Design review of the part shown in the three views and the two pictorial views. Dimensions are in mm from the part's minimum x, y and z. A direction names the side the tool comes from. Give positions to 0.01 mm unless a question says otherwise; leave off trailing zeros. Loops run counter-clockwise (first coordinate to the right, second up) from the corner with the lowest first, then second, coordinate; pieces in that order, holes last. Notation, with made-up numbers: (-2.5, 55.25) - (22.5, 55.25) arc R26 cw to (22.5, 87.25) - close; hole circle Ø1 at (-15, -5.5). An arc over 180 degrees is marked (long way). Return JSON: item names as keys, results as strings. Group by question number.
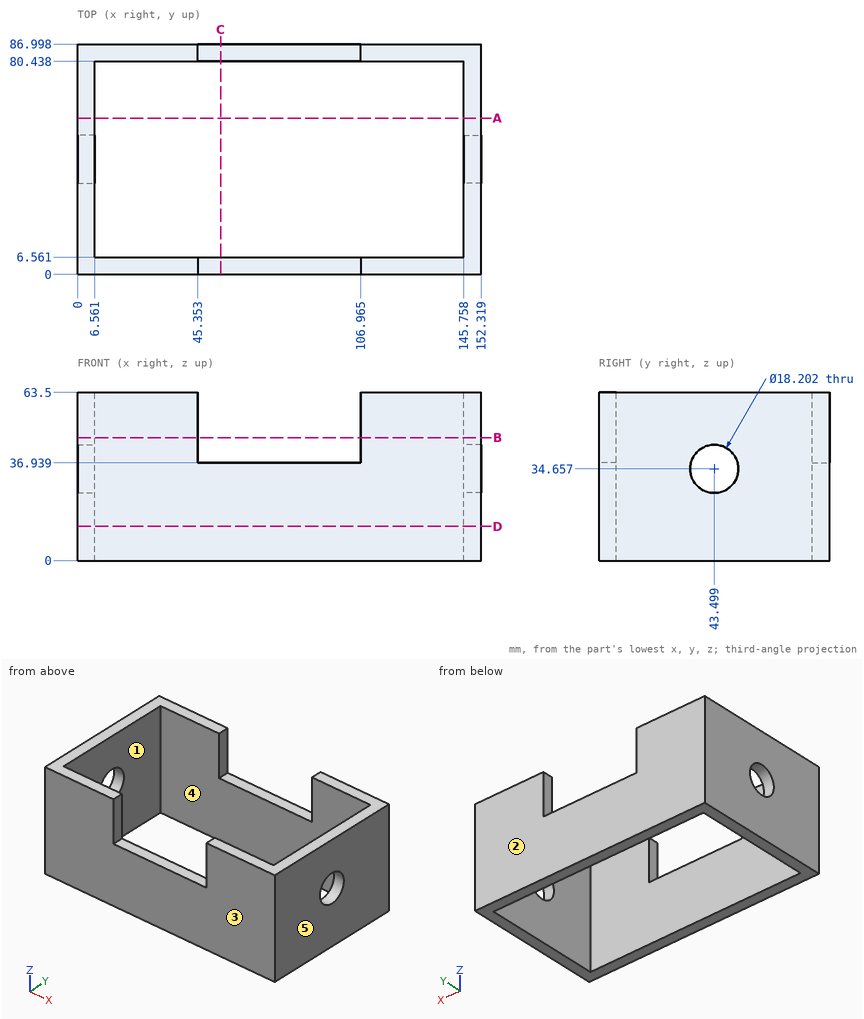
Item 1: Take a section at C-C (x = 54). State the section outline as (y, z) points.
Item 2: Mouldability with a two-part tool opening along Y and no side actions: class the marked faces 1, 2 and 3 as +Y half, -Y half, draft (parallel to the pull), parting line (faces both ways), or undercut.
Item 3: Tool access review of the marked faces 4 and 5: name each direction out of +Z, -Z, +X, -X, +Y, -Y from which nothing blocks a thin tool from reaching the whole face with its end or side.
Item 4: Take a section at B-B (z = 46.5). State the section outline as (x, y) points (1 decimal), then the cut area to 3 significant figures.
Item 5: Take a section at D-D (z = 13). State the section outline as (x, y) points, then the cut area to 3 significant figures.
Item 6: Take a section at A-A (y = 59). State the section outline as (x, z) points, then the cut area to 3 significant figures.
Item 7: For L1, parallel to Y at x = 61, z = 21.5; L2, parallel to X at y = 63, z = 34.5; L3, parallel to Z at x = 60, y = 83, list the stretches that pass through material, from the lowest coordinate up. Write a range as from..to.
Item 8: For P1, Ø10, axis at x = 75, y = 73, coming from the -Z side; P2, Ø5, axis at x = 71.5, y = 2.5, coming from the +Z side, all flat-tipped, find the tip position at first contact; note any pin that passes through.
Check sheet entries:
{
 "1": {"outline": "(0, 0) - (6.56, 0) - (6.56, 36.94) - (0, 36.94) - close; (80.44, 0) - (87, 0) - (87, 36.94) - (80.44, 36.94) - close"},
 "2": {"face 1": "undercut", "face 2": "+Y half", "face 3": "-Y half"},
 "3": {"face 4": "+Z, -Z", "face 5": "+Z, -Z, +X, +Y, -Y"},
 "4": {"outline": "(0, 0) - (45.4, 0) - (45.4, 6.6) - (6.6, 6.6) - (6.6, 80.4) - (45.4, 80.4) - (45.4, 87) - (0, 87) - close; (107, 0) - (152.3, 0) - (152.3, 87) - (107, 87) - (107, 80.4) - (145.8, 80.4) - (145.8, 6.6) - (107, 6.6) - close", "area": "2,160 mm^2"},
 "5": {"outline": "(0, 0) - (152.32, 0) - (152.32, 87) - (0, 87) - close; hole (6.56, 6.56) - (145.76, 6.56) - (145.76, 80.44) - (6.56, 80.44) - close", "area": "2,970 mm^2"},
 "6": {"outline": "(0, 0) - (6.56, 0) - (6.56, 63.5) - (0, 63.5) - close; (145.76, 0) - (152.32, 0) - (152.32, 63.5) - (145.76, 63.5) - close", "area": "833 mm^2"},
 "7": {"L1": "y = 0..6.56, 80.44..87", "L2": "x = 0..6.56, 145.76..152.32", "L3": "z = 0..36.94"},
 "8": {"P1": "passes through", "P2": "stops at z = 36.94"}
}
